Autodesk Inventor part; units mm, degrees
ref_plane "YZ Plane" through (0, 0, 0) normal (1, 0, 0) x (0, 1, 0)
ref_plane "XZ Plane" through (0, 0, 0) normal (0, 1, 0) x (-1, 0, 0)
ref_plane "XY Plane" through (0, 0, 0) normal (0, 0, 1) x (1, 0, 0)
sketch "Sketch1" plane through (0, 0, 0) normal (0, 0, 1) x (1, 0, 0)
  line L0 (-3.3729, 5.842) -> (3.3729, 5.842)
  line L1 (3.3729, 5.842) -> (6.7458, 0)
  line L2 (6.7458, 0) -> (3.3729, -5.842)
  line L3 (3.3729, -5.842) -> (-3.3729, -5.842)
  line L4 (-3.3729, -5.842) -> (-6.7458, 0)
  line L5 (-6.7458, 0) -> (-3.3729, 5.842)
  point P0 (0, 0)
  point P1 (0, 0)
  dimension "d0" = 11.684
extrude "Extrusion1" add sketch "Sketch1" along normal mid plane 2.032
sketch "Sketch2" plane through (0, 0, 0) normal (1, 0, 0) x (0, 1, 0)
  line L0 (5.6521, 1.016) -> (7.9534, 1.016)
  line L1 (7.9534, 1.016) -> (7.9534, 0.3994)
  line L2 (7.9534, 0.3994) -> (5.6521, 1.016)
  line L3 (0, 1.016) -> (5.842, 1.016)
  line L4 (0, -0.4064) -> (0, 2.4384)
  point P0 (0, 0)
  dimension "d3" = 15
revolve "Revolution1" cut sketch "Sketch2" angle 360 about axis through (0, 0, -10) along (0, 0, 1)
mirror "Mirror1" about plane through (0, 0, 0) normal (0, 0, 1) of "Revolution1"
hole "Hole1" at (0, 0, 1.016) direction (0, 0, -1) diameter 9.525 end through all
properties part number "Nut" material "Stainless Steel"
Work out the finished part from the listing and answer in its coordinate system (mm). Round coordinates to 2 decimals unless told otherwise and drop trailing zeros. Order: outer loops, then holes, each group sorted by start corner. A loop starts at its lowest first (then second) coordinate and runs counter-clockwise, first axis right, second up.
Q1. Given pin 1 Ø3 at (x, y) = (1.5, 3.5) entering from -Z; pin 2 Ø1 at (y, z) = (-2.5, 0.5) entering from +X, each flat-ended and moving along its own axis, determine where each tip first touches the part or whether it passes through.
Solution:
pin 1: stops at z = -1.02
pin 2: stops at x = 5.59
Q2. A cutting plane is placed at A-A, the plane x = 0. Determine the outline of the cut face in (y, z).
Solution:
outline: (-5.84, -0.97) - (-5.65, -1.02) - (-4.76, -1.02) - (-4.76, 1.02) - (-5.65, 1.02) - (-5.84, 0.97) - close; (4.76, -1.02) - (5.65, -1.02) - (5.84, -0.97) - (5.84, 0.97) - (5.65, 1.02) - (4.76, 1.02) - close
Q3. A cutting plane is placed at B-B, the plane z = 0.3. Determine the outline of the cut face in (x, y) (1 decimal).
Solution:
outline: (-6.7, 0) - (-3.4, -5.8) - (3.4, -5.8) - (6.7, 0) - (3.4, 5.8) - (-3.4, 5.8) - close; hole circle Ø9.5 at (0, 0)
Q4. The mould has two halves that part along X. Classify faces 1 (the cylindrical face through (2.9, 3.78, -0.01)), 2 (the flat face through (0, -5.842, 0)), 3 (the flat face through (5.083, -2.88, -0.014)): pulls with the +X half, pulls with the -X half, needs draft (parallel to the pull), parting line crosses it, or undercut.
Solution:
face 1: undercut
face 2: needs draft
face 3: pulls with the +X half
Q5. Find the intervals of material crossed by line 1 along Y through (x, z) = (0, 0.55); line 2 along Y through (x, z) = (3, 0.3); line 3 along X through (y, z) = (1, -0.45), in increasing order.
Solution:
line 1: y = -5.84 to -4.76, 4.76 to 5.84
line 2: y = -5.84 to -3.7, 3.7 to 5.84
line 3: x = -6.17 to -4.66, 4.66 to 6.17
